Read the model definition and answer for the solid it produces. Units are mm, in the model's axes. Face numbers are marked on the shaded views. A direction names the side the tool comes from. Round coordinates to 2 decimals unless told otherwise and drop trailing zeros. Write each loop counter-clockwise with the first axis right and the second up, starting at its lowest first coordinate (ties: lowest second). Pieces come first, ordered by that corner, then holes. Notation, with made-up numbers: (50, 15) - (95, 15) arc R6 cw to (95, 21) - close; hole circle Ø1 at (-28.75, 66.5). An arc over 180 degrees is marked (long way). Answer as CSV lines item,"result". Start each with the question number.
1) Which of the six approach directions +Z, -Z, +X, -X, +Y, -Y give full straight-line access (tool end or side, diameter ignored) to the marked faces 1, 2 and 3?
2) Each of these flat-tipped pins is pushed along its axis until it touches: pin 1 (3 mm diameter, centred on x = -27.72, z = 53.97, fed in from +Y); pin 2 (8 mm diameter, centred on y = -8, z = 69.5, fed in from +X); pin 3 (5 mm diameter, centred on y = -1.5, z = -1.5, fed in from -X); pin 4 (5.5 mm diameter, centred on x = -10, z = 35, fed in from -Y). Where does it stop, or does it pass through?
3) Find section B-B on x = 10. Determine the outline of the cut face in (y, z).
4) Find section A-A on z = 35. Determine the outline of the cut face in (x, y).
5) Find section C-C on y = 3. Determine the outline of the cut face in (x, z).
6) Consider line 1 along X through (y, z) = (6.9, 35); line 2 along Y through (x, z) = (-10.5, 24); line 3 along Z through (x, y) = (-0.5, 6.75). Determine where each line is inside the solid, lowest interval first.
7) Find section D-D on x = -5. State how many separate pieces and enclosed holes the cut face has, then the cut area to 3 significant figures.
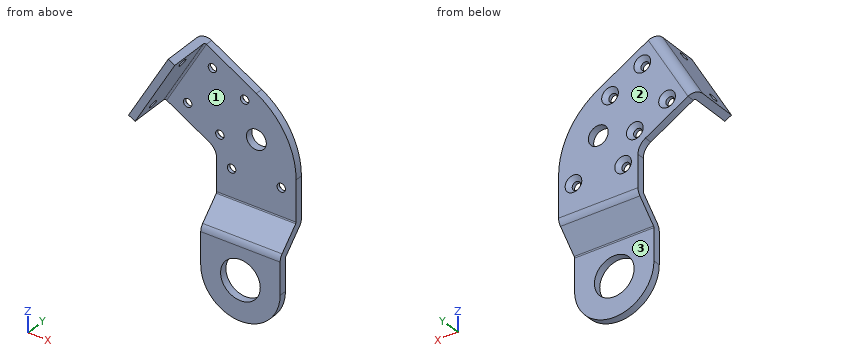
from build123d import *

# Parameters (mm, degrees)
SKETCH2_R                                            = 8
BASE_FLANGE1_DEPTH                                   = 3
EDGE_FLANGE1_START                                   = -16
EDGE_FLANGE1_DEPTH                                   = 32
EDGE_FLANGE1_2_DEPTH                                 = 32
EDGE_FLANGE2_START                                   = -16
EDGE_FLANGE2_DEPTH                                   = 32
EDGE_FLANGE2_2_DEPTH                                 = 32
SKETCH15_R                                           = 4
BOSS_EXTRUDE1_DEPTH                                  = 3
EDGE_FLANGE3_STRIP_W                                 = 13.4732
EDGE_FLANGE3_STRIP_H                                 = 3
EDGE_FLANGE3_STRIP_CUT_DEPTH                         = 32
EDGE_FLANGE3_DEPTH                                   = 32
CSK_FOR_M3_HEX_SOCKET_COUNTERSUNK_CAP_SC_D           = 3.4
CSK_FOR_M3_HEX_SOCKET_COUNTERSUNK_CAP_SC_CSINK_D     = 6.72
CSK_FOR_M3_HEX_SOCKET_COUNTERSUNK_CAP_SC_CSINK_ANGLE = 90
FILLET1_R                                            = 6
M3_CLEARANCE_HOLE1_D                                 = 3.4


# Read off the part's stored shape, not the designer's step: Edge-Flange1, Edge-Flange2
# Sheet-metal steps are written as plain solids
with BuildPart() as part:
    # Sketch2 → Base-Flange1 (new body)
    with BuildSketch(Plane(origin=(0, 0, 0), x_dir=(1, 0, 0), z_dir=(0, 1, 0))):
        with BuildLine():
            Line((-16, 0), (-16, -17.5))
            Line((-16, -17.5), (16, -17.5))
            Line((16, -17.5), (16, 0))
            ThreePointArc((16, 0), (0, 16), (-16, 0))
        make_face()
        with Locations(Location((0, 0, 0), (0, 0, 270))):
            Circle(SKETCH2_R, mode=Mode.SUBTRACT)
    extrude(amount=-BASE_FLANGE1_DEPTH)

    # Edge-Flange1 outline → Edge-Flange1 (cut)
    with BuildSketch(Plane.YZ.offset(EDGE_FLANGE1_START)):
        with BuildLine():
            ThreePointArc((-3, 12.952249603), (-2.715568261, 14.382184516), (-1.905575199, 15.594424801))
            Line((-1.905575199, 15.594424801), (0, 17.5))
            Line((0, 17.5), (-3, 17.5))
            Line((-3, 17.5), (-3, 12.952249603))
        make_face()
    extrude(amount=EDGE_FLANGE1_DEPTH, mode=Mode.SUBTRACT)

    # Edge-Flange1 2 outline → Edge-Flange1 2 (add)
    with BuildSketch(Plane.YZ.offset(EDGE_FLANGE1_START)):
        with BuildLine():
            Line((9.02081528, 26.52081528), (0, 17.5))
            Line((0, 17.5), (0, 12.952249603))
            ThreePointArc((0, 12.952249603), (0.056070336, 13.234134219), (0.215745145, 13.473104458))
            Line((0.215745145, 13.473104458), (11.142135624, 24.399494937))
            Line((11.142135624, 24.399494937), (9.02081528, 26.52081528))
        make_face()
    extrude(amount=EDGE_FLANGE1_2_DEPTH)

    # Edge-Flange2 outline → Edge-Flange2 (cut)
    with BuildSketch(Plane.YZ.offset(EDGE_FLANGE2_START)):
        with BuildLine():
            Line((9.02081528, 26.52081528), (9.02081528, 23.82592499))
            ThreePointArc((9.02081528, 23.82592499), (8.736383541, 22.395990077), (7.926390479, 21.183749792))
            Line((7.926390479, 21.183749792), (11.142135624, 24.399494937))
            Line((11.142135624, 24.399494937), (9.02081528, 26.52081528))
        make_face()
    extrude(amount=EDGE_FLANGE2_DEPTH, mode=Mode.SUBTRACT)

    # Edge-Flange2 2 outline → Edge-Flange2 2 (add)
    with BuildSketch(Plane.YZ.offset(EDGE_FLANGE2_START)):
        with BuildLine():
            Line((5.805070135, 23.305070135), (9.02081528, 26.52081528))
            Line((9.02081528, 26.52081528), (9.02081528, 40.278174593))
            Line((9.02081528, 40.278174593), (6.02081528, 40.278174593))
            Line((6.02081528, 40.278174593), (6.02081528, 23.82592499))
            ThreePointArc((6.02081528, 23.82592499), (5.964744944, 23.544040374), (5.805070135, 23.305070135))
        make_face()
    extrude(amount=EDGE_FLANGE2_2_DEPTH)

    # Sketch15 → Boss-Extrude1 (add)
    with BuildSketch(Plane(origin=(0, 9.02081528, 0), x_dir=(1, 0, 0), z_dir=(0, 1, 0))):
        with BuildLine():
            Line((-16, -40.278174593), (-36.784609691, -52.278174593))
            Line((-36.784609691, -52.278174593), (-20.784609691, -79.990987514))
            Line((-20.784609691, -79.990987514), (0, -67.990987514))
            ThreePointArc((0, -67.990987514), (11.712812921, -56.278174593), (16, -40.278174593))
            Line((16, -40.278174593), (-16, -40.278174593))
        make_face()
        with Locations(Location((0, -50, 0), (0, 0, 270))):
            Circle(SKETCH15_R, mode=Mode.SUBTRACT)
    extrude(amount=-BOSS_EXTRUDE1_DEPTH)

    # Edge-Flange3 strip (across the edge) → Edge-Flange3 strip cut (cut)
    with BuildSketch(Plane(origin=(-20.784609691, 6.02081528, 79.990987514), x_dir=(0.8660254037844396, -3.491481338843133e-15, -0.4999999999999983), z_dir=(-0.4999999999999983, 0, -0.8660254037844396))):
        with Locations((-6, -1.5)):
            Rectangle(EDGE_FLANGE3_STRIP_W, EDGE_FLANGE3_STRIP_H)
    extrude(amount=EDGE_FLANGE3_STRIP_CUT_DEPTH, mode=Mode.SUBTRACT)

    # Edge-Flange3 section (across the edge) → Edge-Flange3 (add)
    with BuildSketch(Plane(origin=(-20.784609691, 6.02081528, 79.990987514), x_dir=(0.8660254037844396, -3.491481338843133e-15, -0.4999999999999983), z_dir=(-0.4999999999999983, 0, -0.8660254037844396))):
        with BuildLine():
            Line((-3, 0.7366), (-3, 17))
            Line((-3, 17), (0, 17))
            Line((0, 17), (0, 0.7366))
            ThreePointArc((0, 0.7366), (0.215745145, 0.215745145), (0.7366, 0))
            Line((0.7366, 0), (0.7366, -3))
            ThreePointArc((0.7366, -3), (-1.905575199, -1.905575199), (-3, 0.7366))
        make_face()
    extrude(amount=EDGE_FLANGE3_DEPTH)

    # CSK for M3 Hex Socket Countersunk Cap Screw1 (through all)
    with Locations(Plane(origin=(0, 9.02081528, 0), x_dir=(1, 0, 0), z_dir=(0, 1, 0))):
        with Locations((-27.722431864, -53.974327016), (-14.732050808, -46.474327016), (-4.732050808, -63.794835091), (-17.722431864, -71.294835091), (-10, -35), (10, -35)):
            CounterSinkHole(CSK_FOR_M3_HEX_SOCKET_COUNTERSUNK_CAP_SC_D / 2, CSK_FOR_M3_HEX_SOCKET_COUNTERSUNK_CAP_SC_CSINK_D / 2, counter_sink_angle=CSK_FOR_M3_HEX_SOCKET_COUNTERSUNK_CAP_SC_CSINK_ANGLE)

    # Fillet1
    fillet1_edges = [part.edges().sort_by_distance(p)[0] for p in [
        (-16, 7.52081528, 40.278174593),
    ]]
    fillet(fillet1_edges, radius=FILLET1_R)

    # M3 Clearance Hole1 (through all)
    with Locations(Plane(origin=(-50.225570899, 0, 28.997746879), x_dir=(-0.49999999999999806, 2.339652494442703e-15, -0.8660254037844398), z_dir=(0.8660254037844397, -4.052396992430042e-15, -0.499999999999998))):
        with Locations((-55.127433482, -3.97918472), (-31.475106897, -3.97918472)):
            Hole(M3_CLEARANCE_HOLE1_D / 2)


solid = part.part
Check values:
1,face 1,"+X, -Y"
1,face 2,"+Z, -Z, +X, -X, +Y"
1,face 3,"-Z, +X, -X, +Y"
2,pin 1,"passes through"
2,pin 2,"stops at x = -24.53"
2,pin 3,"stops at x = -16"
2,pin 4,"stops at y = 6.02"
3,outline,"(-3, -12.49) - (0, -12.49) - (0, 12.95) arc R0.74 cw to (0.22, 13.47) - (7.93, 21.18) arc R3.74 ccw to (9.02, 23.83) - (9.02, 31.64) - (7.36, 33.3) - (6.02, 33.3) - (6.02, 23.83) arc R0.74 cw to (5.81, 23.31) - (-1.91, 15.59) arc R3.74 ccw to (-3, 12.95) - close; (6.02, 36.7) - (7.36, 36.7) - (9.02, 38.36) - (9.02, 58.93) - (6.02, 58.93) - close"
4,outline,"(-16, 6.02) - (-11.7, 6.02) - (-11.7, 7.36) - (-13.36, 9.02) - (-16, 9.02) - close; (-8.3, 6.02) - (8.3, 6.02) - (8.3, 7.36) - (6.64, 9.02) - (-6.64, 9.02) - (-8.3, 7.36) - close; (11.7, 6.02) - (16, 6.02) - (16, 9.02) - (13.36, 9.02) - (11.7, 7.36) - close"
5,outline,"(-39.38, 53.78) - (-36.78, 52.28) - (-20.78, 79.99) - (-23.38, 81.49) - close; (-16, 16.26) - (16, 16.26) - (16, 20.5) - (-16, 20.5) - close"
6,line 1,"x = -16 to -11.7, -8.3 to 8.3, 11.7 to 16"
6,line 2,"y = 6.02 to 9.02"
6,line 3,"z = 20.01 to 46.03, 53.97 to 68.28"
7,separate pieces,"3"
7,enclosed holes,"0"
7,area,"219 mm^2"
